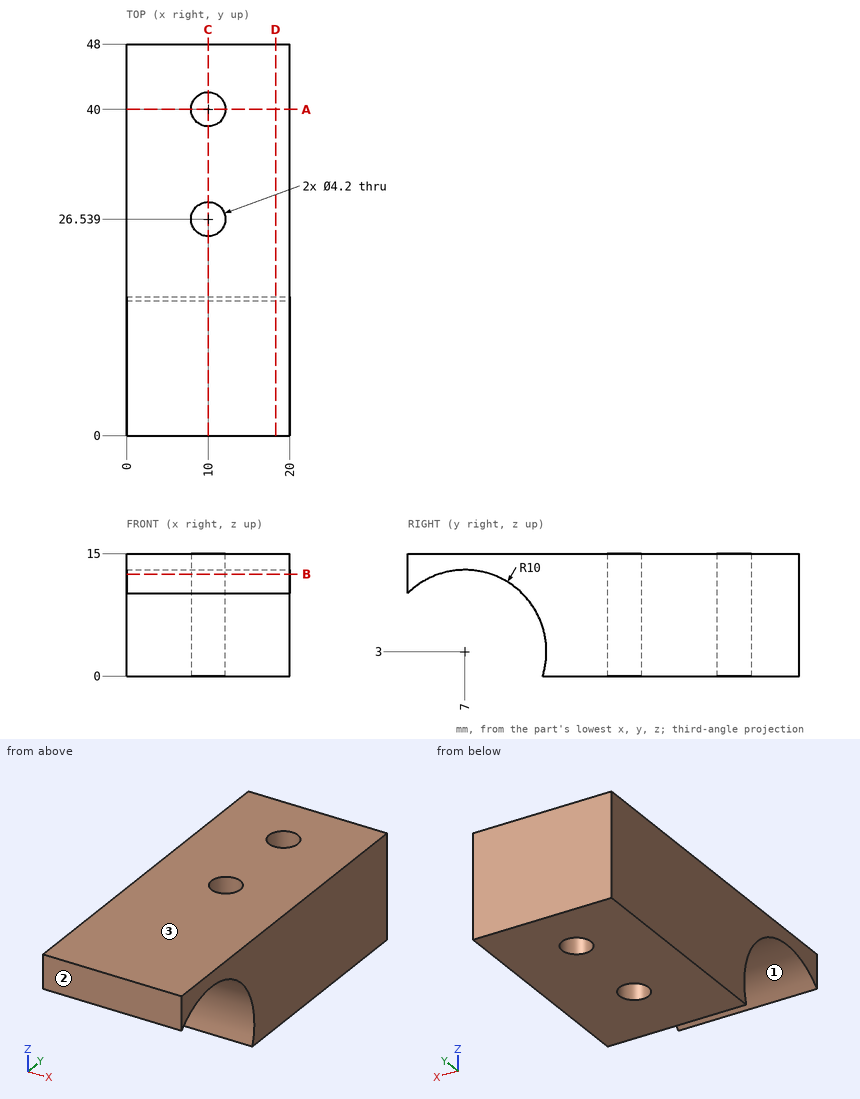
Print and shaded views of the part. All mm, measured from the part's lowest x, y and z. Coordinates: 2 decimals unless noted, no trailing zeros. Write each loop counter-clockwise with the first axis right and the second up, starting at its lowest first coordinate (ties: lowest second). Pieces come first, ordered by that corner, then holes. Notation, with made-up numbers: (-35, -38.75) - (-13, -38.75) arc R29 cw to (-13, -5.75) - close; hole circle Ø6 at (30.25, 21). An arc over 180 degrees is marked (long way). One line per question, with ' | ' between items. Start each with the question number.
Q1. Cut at B-B, the plane z = 12.5. List the corners of the cut face in (x, y).
Q2. Cut at C-C, the plane x = 10. List the corners of the cut face in (y, z), then the cut area to 3 significant figures.
Q3. Pull direction Y, two halves, no side cores. Call the marked faces 1, 2 and 3: pulls with the +Y half, pulls with the -Y half, needs draft (parallel to the pull), parting line crosses it, or undercut.
Q4. Cut at A-A, the plane y = 40. List the corners of the cut face in (x, z), then the cut area to 3 significant figures.
Q5. Pin check, flat tips, straight feed: pin 1 (6 mm diameter, centred on x = 13.5, y = 11, fed in from -Z); pin 2 (1.5 mm diameter, centred on x = 7, z = 2, fed in from -Y). Stop position of each tip, or through.
Q6. Drill centre lines: line 1 (Y direction, x = 9.5, z = 14.75); line 2 (Y direction, x = 9.5, z = 11.25); line 3 (Y direction, x = 10, z = 6.5). Where is each one in solid material? Low to high. Write a range as [from, to].
Q7. Cut at D-D, the plane x = 18.25. List the corners of the cut face in (y, z), then the cut area to 3 significant figures.
Answer below:
1) outline: (0, 0) - (20, 0) - (20, 3.88) - (0, 3.88) - close; (0, 10.12) - (20, 10.12) - (20, 48) - (0, 48) - close; hole circle Ø4.2 at (10, 26.54); hole circle Ø4.2 at (10, 40)
2) outline: (0, 10.14) arc R10 cw to (16.54, 0) - (24.44, 0) - (24.44, 15) - (0, 15) - close; (28.64, 0) - (37.9, 0) - (37.9, 15) - (28.64, 15) - close; (42.1, 0) - (48, 0) - (48, 15) - (42.1, 15) - close | area: 401 mm^2
3) face 1: undercut | face 2: pulls with the -Y half | face 3: needs draft
4) outline: (0, 0) - (7.9, 0) - (7.9, 15) - (0, 15) - close; (12.1, 0) - (20, 0) - (20, 15) - (12.1, 15) - close | area: 237 mm^2
5) pin 1: z = 10.14 | pin 2: y = 16.85
6) line 1: [0, 24.5], [28.58, 37.96], [42.04, 48] | line 2: [0, 1.35], [12.65, 24.5], [28.58, 37.96], [42.04, 48] | line 3: [16.37, 24.44], [28.64, 37.9], [42.1, 48]
7) outline: (0, 10.14) arc R10 cw to (16.54, 0) - (48, 0) - (48, 15) - (0, 15) - close | area: 527 mm^2
